Model file for the job. Use its own axes, mm. A direction names the side the tool comes from. Give positions to 0.01 mm unless a question says otherwise; leave off trailing zeros. Write each loop counter-clockwise with the first axis right and the second up, starting at its lowest first coordinate (ties: lowest second). Pieces come first, ordered by that corner, then holes.
```python
from build123d import *

# Parameters (mm, degrees)
F1_DEPTH = 27.94
F2_R     = 9.779
F3_DEPTH = 2
F5_DEPTH = 25.4


with BuildPart() as f1:
    # F0 (on Right) → F1 (new body)
    with BuildSketch(Plane.YZ):
        Polygon((0, 12.7), (0, 0), (50.8, 0), (76.2, 12.7), align=None)
    extrude(amount=F1_DEPTH)

    # F2 (on face) → F3 (cut)
    with BuildSketch(Plane.XY.offset(12.7)):
        with Locations((13.97, 38.227)):
            Circle(F2_R)
    extrude(amount=-F3_DEPTH, mode=Mode.SUBTRACT)

    # F4 (on Top) → F5 (cut)
    with BuildSketch(Plane.XY):
        with BuildLine():
            ThreePointArc((0, 44.323), (-6.35, 37.973), (0, 31.623))
            Line((0, 31.623), (0, 37.973))
            Line((0, 37.973), (0, 44.323))
        make_face()
        with BuildLine():
            Line((0, 37.973), (0, 31.623))
            ThreePointArc((0, 31.623), (4.490128, 33.482872), (6.35, 37.973))
            Line((6.35, 37.973), (0, 37.973))
        make_face()
        with BuildLine():
            Line((0, 44.323), (0, 37.973))
            Line((0, 37.973), (6.35, 37.973))
            ThreePointArc((6.35, 37.973), (4.490128, 42.463128), (0, 44.323))
        make_face()
    extrude(amount=F5_DEPTH, mode=Mode.SUBTRACT)


solid = f1.part
```
1. Pin check, flat tips, straight feed: P1, Ø1.5, axis at y = 61.5, z = 4, coming from the -X side; P2, Ø4, axis at x = 9, z = 8.5, coming from the +Y side; P3, Ø1.5, axis at x = 4, z = 2.5, coming from the +Y side; P4, Ø5, axis at x = 17.5, y = 34.5, coming from the +Z side. Stop position of each tip, or through.
Calculated:
P1: passes through
P2: stops at y = 71.8
P3: stops at y = 57.3
P4: stops at z = 10.7
2. Pull direction X, two halves, no side cores. Call faces 1 (the flat face through (27.94, 29, 6)), 2 (the flat face through (14, 38, 10.7)), 3 (the flat face through (20, 47, 12.7)): +X half, -X half, draft (parallel to the pull), parting line (faces both ways), or undercut.
Calculated:
face 1: +X half
face 2: undercut
face 3: draft
3. Slice it at A-A, the plane z = 8. Write the cut outline in (x, y).
Calculated:
outline: (0, 0) - (27.94, 0) - (27.94, 66.8) - (0, 66.8) - (0, 44.32) arc R6.35 cw to (0, 31.62) - close
4. Slice it at D-D, the plane x = 25.25. Write the cut outline in (y, z), and give its area (3 significant figures).
Calculated:
outline: (0, 0) - (50.8, 0) - (76.2, 12.7) - (0, 12.7) - close
area: 806 mm2
5. Slice it at B-B, the plane x = 13.97. Write the cut outline in (y, z).
Calculated:
outline: (0, 0) - (50.8, 0) - (76.2, 12.7) - (48.01, 12.7) - (48.01, 10.7) - (28.45, 10.7) - (28.45, 12.7) - (0, 12.7) - close
6. Slice it at C-C, the plane y = 67. Write the cut outline in (x, z).
Calculated:
outline: (0, 8.1) - (27.94, 8.1) - (27.94, 12.7) - (0, 12.7) - close
7. Probe probe 1 along Y at (x, z) = (13.97, 11.3); probe 2 along Y at (x, z) = (2, 10.5); probe 3 along Y at (x, z) = (23.25, 7.5). List the from-to ranges inside material, lowest first.
Calculated:
probe 1: y = 0 to 28.45, 48.01 to 73.4
probe 2: y = 0 to 31.95, 44 to 71.8
probe 3: y = 0 to 65.8
8. Which spindle directions (+Z, -Z, +X, -X, +Y, -Y) get a long thin tool onto all of the face, cutting with end or side? Do faces 4 (the flat face through (13.77, 63.32, 6.26)), 5 (the cylindrical face through (23.747, 38.031, 11.714)). Say none if no direction does.
Calculated:
face 4: -Z, +X, -X, +Y
face 5: +Z
